Here's how the part is built. I have some questions about the finished solid (model axes, mm). A direction names the side the tool comes from. Give positions to 0.01 mm unless a question says otherwise; leave off trailing zeros. Write each loop counter-clockwise with the first axis right and the second up, starting at its lowest first coordinate (ties: lowest second). Pieces come first, ordered by that corner, then holes. Notation, with made-up numbers: M 0,59.25 L 13,59.25 A9 cw 13,66.25 Z; hole C 6.5,48 d2. An arc over 180 degrees is marked long. Use one line per item in the form item = value. Start each with the question number.
Autodesk Inventor part; units mm, degrees
ref_plane "YZ Plane" through (0, 0, 0) normal (1, 0, 0) x (0, 1, 0)
ref_plane "XZ Plane" through (0, 0, 0) normal (0, 1, 0) x (-1, 0, 0)
ref_plane "XY Plane" through (0, 0, 0) normal (0, 0, 1) x (1, 0, 0)
sketch "Sketch1" plane through (0, 0, 0) normal (0, 1, 0) x (-1, 0, 0)
  line L0 (-2.875, 6.65) -> (2.875, 6.65)
  line L1 (2.875, 6.65) -> (2.875, -6.65)
  line L2 (2.875, -6.65) -> (-2.875, -6.65)
  line L3 (-2.875, -6.65) -> (-2.875, 6.65)
  line L4 (-2.875, 6.65) -> (2.875, -6.65) construction
  line L5 (2.875, 6.65) -> (-2.875, -6.65) construction
  line L6 (2.475, -6.25) -> (2.475, 6.25)
  line L7 (2.475, 6.25) -> (-2.475, 6.25)
  line L8 (-2.475, 6.25) -> (-2.475, -6.25)
  line L9 (-2.475, -6.25) -> (2.475, -6.25)
  circle A0 centre (1.285, 3.81) radius 0.5
  point P0 (0, 0)
  dimension "d0" = 13.3
  dimension "d1" = 5.75
  dimension "d2" = 0.4
  dimension "d7" = 1
  dimension "d8" = 4.16
  dimension "d9" = 3.81
extrude "Extrusion1" add sketch "Sketch1" along normal blind 14.9 contours L0 L1 L2 L3
extrude "Extrusion2" add sketch "Sketch1" along normal blind 0.4 contours L9 L8 L7 L6 | A0
extrude "Extrusion3" add sketch "Sketch1" against normal blind 2 contours A0
pattern_linear "Rectangular Pattern1" count 4 spacing 2.54 along (0, 0, -1) of "Extrusion3"
properties part number "Female USB SMT"
1) Suppose I cut it at C-C, the plane z = 1.27. List the corners of the cut face in (x, y) for me (3 decimals).
2) Suppose I cut it at A-A, the plane y = 5.25. List the corners of the cut face in (x, z) for me (3 decimals), and give its area (3 significant figures).
3) Will this pin go through, and if not, where does the flat tip stop? P1, Ø1, axis at x = 1, z = 3.5, coming from the -Y side.
4) On a 3-axis mill with a long thin cutter (end or side, diameter ignored), from which of +Z, -Z, +X, -X, +Y, -Y can I reach the whole of each face in a straight line? I mean faces 4 (the face through (-1.22, -0.986, -3.314)), 5 (the face through (0, 7, 6.65)), 6 (the face through (0, 8, -6.25)). Say none if no direction works.
5) Suppose I cut it at B-B, the plane x = 0.2. List the corners of the cut face in (y, z) for me, and give its area (3 significant figures).
6) Thinking about a two-plate mould opening in X: for faces 1 (the face through (-1.3, -2, -1.3)), 2 (the face through (0, 8, 6.25)), 3 (the face through (-1.554, -0.986, 1.692)), which applies, released by +X, released by -X, zero draft, split by the parting line, or undercut?
7) Suppose I cut it at D-D, the plane y = -1. List the corners of the cut face in (x, z) for me (3 decimals).
8) Please list where these lines run through material, in increasing order: line 1 (X direction, y = 2, z = 3.5) (3 decimals); line 2 (Z direction, x = 1.35, y = 10.75); line 3 (Y direction, x = -2.2, z = -1).
Checks:
q1.outline = M -2.875,0 L -1.785,0 L -1.785,-2 L -0.785,-2 L -0.785,0 L 2.875,0 L 2.875,14.9 L 2.475,14.9 L 2.475,0.4 L -2.475,0.4 L -2.475,14.9 L -2.875,14.9 Z
q2.outline = M -2.875,-6.65 L 2.875,-6.65 L 2.875,6.65 L -2.875,6.65 Z; hole M -2.475,-6.25 L 2.475,-6.25 L 2.475,6.25 L -2.475,6.25 Z
q2.area = 14.6 mm^2
q3.P1 = 0
q4.face_4 = -Y
q4.face_5 = +Z, +X, -X, +Y, -Y
q4.face_6 = +Y
q5.outline = M 0,-6.65 L 14.9,-6.65 L 14.9,-6.25 L 0.4,-6.25 L 0.4,6.25 L 14.9,6.25 L 14.9,6.65 L 0,6.65 Z
q5.area = 16.9 mm^2
q6.face_1 = zero draft
q6.face_2 = undercut
q6.face_3 = split by the parting line
q7.outline = C -1.285,-3.81 d1; C -1.285,-1.27 d1; C -1.285,1.27 d1; C -1.285,3.81 d1
q8.line_1 = -2.875 to -2.475, 2.475 to 2.875
q8.line_2 = -6.65 to -6.25, 6.25 to 6.65
q8.line_3 = 0 to 0.4
